Here's how the part is built. I have some questions about the finished solid (model axes, mm). A direction names the side the tool comes from. Coordinates: 2 decimals unless noted, no trailing zeros. Write each loop counter-clockwise with the first axis right and the second up, starting at its lowest first coordinate (ties: lowest second). Pieces come first, ordered by that corner, then holes. Notation, with made-up numbers: M 71.25,77 L 78.25,77 A20 cw 78.25,82 Z; hole C 14,60 d3. An arc over 180 degrees is marked long. Use one line per item in the form item = value. Start each with the question number.
1. I want a section at A-A, the plane x = -31. List the corners of the cut face in (y, z) for me, plus the area to 3 significant figures.
2. I want a section at C-C, the plane z = -42.5. List the corners of the cut face in (x, y) for me.
3. On a 3-axis mill with a long thin cutter (end or side, diameter ignored), from which of +Z, -Z, +X, -X, +Y, -Y can I reach the whole of each face in a straight line? I mean faces 1 (the face through (-78, 1, 4)), 2 (the face through (-120, 1, -11)), 3 (the face through (53, 1, -53)), 4 (the face through (-78, 1, -55)). Say none if no direction works.
4. I want a section at D-D, the plane x = -66.5. List the corners of the cut face in (y, z) for me.
5. I'm going to push flat-ended pins straight in: pin 1 Ø8 at (x, z) = (-58, -34) entering from +Y; pin 2 Ø1.5 at (y, z) = (2, -34.5) entering from -X; pin 3 Ø0.9 at (y, z) = (2, -54) entering from -X; pin 4 Ø0.9 at (y, z) = (1.5, -43) entering from +X. Where does each tip first touch, or does it pass through?
6. Thinking about a two-plate mould opening in Z: for faces 5 (the face through (-120, 1, -41)), 6 (the face through (-122.176, 1.479, -2.412)), 7 (the face through (29, 1, 3)), which applies, released by +Z, released by -Z, zero draft, split by the parting line, or undercut?
7. I want a section at B-B, the plane z = -25.5. List the corners of the cut face in (x, y) for me, plus the area to 3 significant figures.
8. Please list where these lines run through material, in increasing order: line 1 along Z through (x, y) = (-31, 1.9); line 2 along Z through (x, y) = (-67, 2.65); line 3 along X through (y, z) = (1.95, 2.5). Write a range as [from, to].
Autodesk Inventor part; units mm, degrees
ref_plane "YZ Plane" through (0, 0, 0) normal (1, 0, 0) x (0, 1, 0)
ref_plane "XZ Plane" through (0, 0, 0) normal (0, 1, 0) x (-1, 0, 0)
ref_plane "XY Plane" through (0, 0, 0) normal (0, 0, 1) x (1, 0, 0)
sketch "Sketch1" plane through (0, 0, 0) normal (0, 1, 0) x (-1, 0, 0)
  line L0 (37.5, -2) -> (24.5, -2) construction
  line L1 (24.5, -2) -> (24.5, -15) construction
  line L2 (24.5, -15) -> (37.5, -15) construction
  line L3 (37.5, -15) -> (37.5, -2) construction
  line L4 (56.9183, -8.5) -> (8.3915, -8.5) construction
  line L5 (0, -17) -> (105, -17) construction
  line L6 (0, 0) -> (0, -51) construction
  line L7 (0, -34) -> (105, -34) construction
  line L8 (105, -51) -> (105, 0) construction
  line L9 (31, 55.8243) -> (31, -51) construction
  line L10 (56.8064, -25.5) -> (17, -25.5) construction
  line L11 (24.5, -19) -> (24.5, -32) construction
  line L12 (37.5, -19) -> (24.5, -19) construction
  line L13 (37.5, -32) -> (37.5, -19) construction
  line L14 (24.5, -32) -> (37.5, -32) construction
  line L15 (24.5, -36) -> (24.5, -49) construction
  line L16 (37.5, -36) -> (24.5, -36) construction
  line L17 (37.5, -49) -> (37.5, -36) construction
  line L18 (24.5, -49) -> (37.5, -49) construction
  line L19 (56.3008, -42.5) -> (16.5498, -42.5) construction
  arc A0 (50, -12) -> (50, -22) centre (50, -17) ccw
  arc A1 (91, -22) -> (91, -12) centre (91, -17) ccw
  arc A2 (50, -29) -> (50, -39) centre (50, -34) ccw
  arc A3 (91, -39) -> (91, -29) centre (91, -34) ccw
  line L20 (50, -12) -> (91, -12)
  line L21 (50, -22) -> (91, -22)
  line L22 (50, -29) -> (91, -29)
  line L23 (50, -39) -> (91, -39)
  arc A4 (14.45, -38) -> (14.45, -30) centre (14.45, -34) ccw
  line L24 (103.5, -49.5) -> (103.5, -1.5) construction
  line L25 (1.5, -1.5) -> (1.5, -49.5) construction
  arc A5 (14, -30) -> (14, -38) centre (14, -34) ccw
  arc A6 (14, -13) -> (14, -21) centre (14, -17) ccw
  line L26 (14.45, -38) -> (14, -38)
  line L27 (14, -30) -> (14.45, -30)
  line L28 (14, -21) -> (14.45, -21)
  line L29 (14.45, -13) -> (14, -13)
  arc A7 (14.45, -21) -> (14.45, -13) centre (14.45, -17) ccw
  arc A8 (96.5, -51) -> (93, -47.5) centre (93, -51) ccw construction
  arc A9 (50, -47.5) -> (46.5, -51) centre (50, -51) ccw construction
  arc A10 (97.7697, -49.5) -> (93, -46) centre (93, -51) ccw construction
  line L30 (93, -46) -> (50, -46) construction
  line L31 (96.5, -51) -> (105, -51) construction
  line L32 (93, -47.5) -> (50, -47.5) construction
  line L33 (105, -49.5) -> (97.7697, -49.5) construction
  arc A11 (50, -46) -> (45.2303, -49.5) centre (50, -51) ccw construction
  arc A12 (45.2303, -1.5) -> (50, -5) centre (50, 0) ccw construction
  arc A13 (46.5, 0) -> (50, -3.5) centre (50, 0) ccw construction
  line L34 (93, -3.5) -> (50, -3.5) construction
  line L35 (93, -5) -> (50, -5) construction
  line L36 (97.7697, -1.5) -> (105, -1.5) construction
  line L37 (105, 0) -> (96.5, 0) construction
  arc A14 (93, -3.5) -> (96.5, 0) centre (93, 0) ccw construction
  arc A15 (93, -5) -> (97.7697, -1.5) centre (93, 0) ccw construction
  arc A16 (17.95, -51) -> (14.45, -47.5) centre (14.45, -51) ccw construction
  arc A17 (12, -47.5) -> (8.5, -51) centre (12, -51) ccw construction
  line L38 (14.45, -46) -> (12, -46) construction
  line L39 (14.45, -47.5) -> (12, -47.5) construction
  arc A18 (12, -46) -> (7.2303, -49.5) centre (12, -51) ccw construction
  arc A19 (19.2197, -49.5) -> (14.45, -46) centre (14.45, -51) ccw construction
  line L40 (45.2303, -49.5) -> (19.2197, -49.5) construction
  line L41 (7.2303, -49.5) -> (0, -49.5) construction
  line L42 (0, -51) -> (8.5, -51) construction
  line L43 (17.95, -51) -> (46.5, -51) construction
  line L44 (14.45, -5) -> (12, -5) construction
  line L45 (14.45, -3.5) -> (12, -3.5) construction
  arc A20 (8.5, 0) -> (12, -3.5) centre (12, 0) ccw construction
  arc A21 (14.45, -3.5) -> (17.95, 0) centre (14.45, 0) ccw construction
  arc A22 (7.2303, -1.5) -> (12, -5) centre (12, 0) ccw construction
  arc A23 (14.45, -5) -> (19.2197, -1.5) centre (14.45, 0) ccw construction
  line L46 (46.5, 0) -> (17.95, 0) construction
  line L47 (8.5, 0) -> (0, 0) construction
  line L48 (0, -1.5) -> (7.2303, -1.5) construction
  line L49 (19.2197, -1.5) -> (45.2303, -1.5) construction
  arc A24 (39, -4) -> (35.5, -0.5) centre (35.5, -4) ccw construction
  arc A25 (26.5, -0.5) -> (23, -4) centre (26.5, -4) ccw construction
  arc A26 (35.5, -50.5) -> (39, -47) centre (35.5, -47) ccw construction
  arc A27 (23, -47) -> (26.5, -50.5) centre (26.5, -47) ccw construction
  line L50 (39, -4) -> (39, -47) construction
  line L51 (35.5, -0.5) -> (26.5, -0.5) construction
  line L52 (23, -4) -> (23, -47) construction
  line L53 (26.5, -50.5) -> (35.5, -50.5) construction
  line L54 (51, 5) -> (51, 2)
  line L55 (78, 5) -> (78, 2)
  line L56 (94, 5) -> (94, 2)
  line L57 (11, 5) -> (11, 2)
  line L58 (-29, 2) -> (-29, 5)
  line L59 (51, -56) -> (51, -53)
  line L60 (11, -56) -> (11, -53)
  line L61 (-29, -56) -> (-29, -53)
  line L62 (78, -56) -> (78, -53)
  line L63 (94, -56) -> (94, -53)
  line L64 (-47, 5) -> (-47, 2)
  line L65 (-47, -53) -> (-47, -56)
  line L66 (11, 2) -> (-29, 2)
  line L67 (120, 2) -> (94, 2)
  line L68 (78, 2) -> (51, 2)
  line L69 (51, -53) -> (78, -53)
  line L70 (94, -53) -> (120, -53)
  line L71 (-29, -53) -> (11, -53)
  line L72 (-47, 2) -> (-59, 2)
  line L73 (-59, -53) -> (-47, -53)
  circle A28 centre (31, -8.5) radius 4
  circle A29 centre (31, -25.5) radius 4
  circle A30 centre (31, -42.5) radius 4
  line L74 (51, 5) -> (11, 5)
  line L75 (-29, 5) -> (-47, 5)
  line L76 (-47, -56) -> (-29, -56)
  line L77 (11, -56) -> (51, -56)
  line L78 (78, -56) -> (94, -56)
  line L79 (-59, 2) -> (-59, -19.5)
  line L80 (-59, -31.5) -> (-59, -53)
  line L81 (120, -5.5) -> (116.8, -5.5)
  line L82 (116.8, -5.5) -> (116.8, -15.5)
  line L83 (116.8, -15.5) -> (120, -15.5)
  line L84 (120, -15.5) -> (120, -5.5)
  line L85 (120, -35.5) -> (116.8, -35.5)
  line L86 (116.8, -35.5) -> (116.8, -45.5)
  line L87 (116.8, -45.5) -> (120, -45.5)
  line L88 (120, -45.5) -> (120, -35.5)
  line L89 (-59, -19.5) -> (-29, -19.5)
  arc A31 (-29, -20.5) -> (-29, -19.5) centre (-29, -20) ccw
  line L90 (-29, -20.5) -> (-62, -20.5)
  line L91 (-62, -30.5) -> (-29, -30.5)
  arc A32 (-29, -31.5) -> (-29, -30.5) centre (-29, -31) ccw
  line L92 (-59, -31.5) -> (-29, -31.5)
  arc A33 (-62, -20.5) -> (-66, -20.5) centre (-64, -20.5) ccw
  arc A34 (-66, -30.5) -> (-62, -30.5) centre (-64, -30.5) ccw
  line L93 (-66, -30.5) -> (-66, -20.5)
  arc A35 (120, -50.8104) -> (123, -45.5) centre (116.8, -45.5) ccw
  arc A36 (123, -5.5) -> (120, -0.1896) centre (116.8, -5.5) ccw
  line L94 (120, -0.1896) -> (120, 2)
  line L95 (120, -50.8104) -> (120, -53)
  arc A37 (123, -35.5) -> (120, -30.1896) centre (116.8, -35.5) ccw
  arc A38 (120, -20.8104) -> (123, -15.5) centre (116.8, -15.5) ccw
  line L96 (120, -20.8104) -> (120, -30.1896)
  line L97 (123, -45.5) -> (123, -35.5)
  line L98 (123, -15.5) -> (123, -5.5)
  line L99 (94, 5) -> (78, 5)
  dimension "d0" = 13
  dimension "d2" = 17
  dimension "d3" = 31
  dimension "d4" = 105
  dimension "d5" = 17
  dimension "d6" = 17
  dimension "d7" = 10
  dimension "d8" = 1.5
  dimension "d9" = 1.5
  dimension "d10" = 4
  dimension "d11" = 1.5
  dimension "d12" = 1.5
  dimension "d13" = 1.5
  dimension "d14" = 17
  dimension "d15" = 17
  dimension "d16" = 12
  dimension "d17" = 14
  dimension "d19" = 12
  dimension "d20" = 2
  dimension "d21" = 2
  dimension "d22" = 7
  dimension "d23" = 2
  dimension "d24" = 2
  dimension "d25" = 40
  dimension "d26" = 40
  dimension "d27" = 18
  dimension "d30" = 2
  dimension "d31" = 14
  dimension "d33" = 19
  dimension "d38" = 55
  dimension "d39" = 8
  dimension "d46" = 3
  dimension "d52" = 12
  dimension "d53" = 10
  dimension "d54" = 3.2
  dimension "d56" = 20
  dimension "d57" = 30
  dimension "d58" = 1
  dimension "d59" = 10
  dimension "d60" = 4
  dimension "d62" = 3
  dimension "d64" = 3
  dimension "d67" = 27
  dimension "d68" = 16
  dimension "d71" = 26
  dimension "d72" = 16.55
extrude "Extrusion1" add sketch "Sketch1" along normal blind 3
properties part number "Bottom_plate2" material "Polycarbonate, Clear"
Answer list:
q1.outline = M 0,-56 L 3,-56 L 3,-46.5 L 0,-46.5 Z; M 0,-38.5 L 3,-38.5 L 3,-29.5 L 0,-29.5 Z; M 0,-21.5 L 3,-21.5 L 3,-12.5 L 0,-12.5 Z; M 0,-4.5 L 3,-4.5 L 3,5 L 0,5 Z
q1.area = 111 mm²
q2.outline = M -123,0 L -120,0 L -120,3 L -123,3 Z; M -116.8,0 L -35,0 L -35,3 L -116.8,3 Z; M -27,0 L 59,0 L 59,3 L -27,3 Z
q3.face_1 = +Z, +Y, -Y
q3.face_2 = +Y, -Y
q3.face_3 = -Z, +X, +Y, -Y
q3.face_4 = -Z, +Y, -Y
q4.outline = M 0,-53 L 3,-53 L 3,-39 L 0,-39 Z; M 0,-29 L 3,-29 L 3,-22 L 0,-22 Z; M 0,-12 L 3,-12 L 3,2 L 0,2 Z
q5.pin_1 = through
q5.pin_2 = -122.99
q5.pin_3 = -94
q5.pin_4 = 59
q6.face_5 = undercut
q6.face_6 = released by +Z
q6.face_7 = zero draft
q7.outline = M -120,0 L -35,0 L -35,3 L -120,3 Z; M -27,0 L 66,0 L 66,3 L -27,3 Z
q7.area = 534 mm²
q8.line_1 = [-56, -46.5], [-38.5, -29.5], [-21.5, -12.5], [-4.5, 5]
q8.line_2 = [-53, -39], [-29, -22], [-12, 2]
q8.line_3 = [-94, -78], [-51, -11], [29, 47]
